from build123d import *

# Parameters (mm, degrees)
SKETCH1_W           = 35
SKETCH1_H           = 35
BOSS_EXTRUDE2_DEPTH = 20
SKETCH2_W           = 35
SKETCH2_H           = 10
BOSS_EXTRUDE3_DEPTH = 20
SKETCH3_W           = 35
SKETCH3_H           = 35
BOSS_EXTRUDE4_DEPTH = 5
CUT_EXTRUDE1_REACH  = 53.357
SKETCH4_R           = 1.5


with BuildPart() as part:
    # Sketch1 → Boss-Extrude2 (new body)
    with BuildSketch(Plane(origin=(0, 0, 0), x_dir=(1, 0, 0), z_dir=(0, 1, 0))):
        Rectangle(SKETCH1_W, SKETCH1_H)
    extrude(amount=BOSS_EXTRUDE2_DEPTH)

    # Sketch2 → Boss-Extrude3 (add)
    with BuildSketch(Plane(origin=(0, 20, 0), x_dir=(1, 0, 0), z_dir=(0, 1, 0))):
        Rectangle(SKETCH2_W, SKETCH2_H)
    extrude(amount=BOSS_EXTRUDE3_DEPTH)

    # Sketch3 → Boss-Extrude4 (add)
    with BuildSketch(Plane(origin=(0, 40, 0), x_dir=(1, 0, 0), z_dir=(0, 1, 0))):
        Rectangle(SKETCH3_W, SKETCH3_H)
    extrude(amount=BOSS_EXTRUDE4_DEPTH)

    # Sketch4 → Cut-Extrude1 (cut, up to next)
    with BuildSketch(Plane(origin=(0, 45, 0), x_dir=(1, 0, 0), z_dir=(0, 1, 0)), mode=Mode.PRIVATE) as cut_extrude1_sk1:
        with Locations(Location((-14.5, 14.5, 0), (0, 0, 270))):
            Circle(SKETCH4_R)
    cut_extrude1_tool1 = extrude(cut_extrude1_sk1.sketch, amount=-CUT_EXTRUDE1_REACH, mode=Mode.PRIVATE) & part.part
    # Sketch4 → Cut-Extrude1 (cut, up to next)
    with BuildSketch(Plane(origin=(0, 45, 0), x_dir=(1, 0, 0), z_dir=(0, 1, 0)), mode=Mode.PRIVATE) as cut_extrude1_sk2:
        with Locations(Location((14.5, 14.5, 0), (0, 0, 270))):
            Circle(SKETCH4_R)
    cut_extrude1_tool2 = extrude(cut_extrude1_sk2.sketch, amount=-CUT_EXTRUDE1_REACH, mode=Mode.PRIVATE) & part.part
    # Sketch4 → Cut-Extrude1 (cut, up to next)
    with BuildSketch(Plane(origin=(0, 45, 0), x_dir=(1, 0, 0), z_dir=(0, 1, 0)), mode=Mode.PRIVATE) as cut_extrude1_sk3:
        with Locations(Location((14.5, -14.5, 0), (0, 0, 270))):
            Circle(SKETCH4_R)
    cut_extrude1_tool3 = extrude(cut_extrude1_sk3.sketch, amount=-CUT_EXTRUDE1_REACH, mode=Mode.PRIVATE) & part.part
    # Sketch4 → Cut-Extrude1 (cut, up to next)
    with BuildSketch(Plane(origin=(0, 45, 0), x_dir=(1, 0, 0), z_dir=(0, 1, 0)), mode=Mode.PRIVATE) as cut_extrude1_sk4:
        with Locations(Location((-14.5, -14.5, 0), (0, 0, 270))):
            Circle(SKETCH4_R)
    cut_extrude1_tool4 = extrude(cut_extrude1_sk4.sketch, amount=-CUT_EXTRUDE1_REACH, mode=Mode.PRIVATE) & part.part
    add(cut_extrude1_tool1.solids().sort_by_distance((-14.5, 45, -14.5))[0], mode=Mode.SUBTRACT)
    add(cut_extrude1_tool2.solids().sort_by_distance((14.5, 45, -14.5))[0], mode=Mode.SUBTRACT)
    add(cut_extrude1_tool3.solids().sort_by_distance((14.5, 45, 14.5))[0], mode=Mode.SUBTRACT)
    add(cut_extrude1_tool4.solids().sort_by_distance((-14.5, 45, 14.5))[0], mode=Mode.SUBTRACT)


solid = part.part
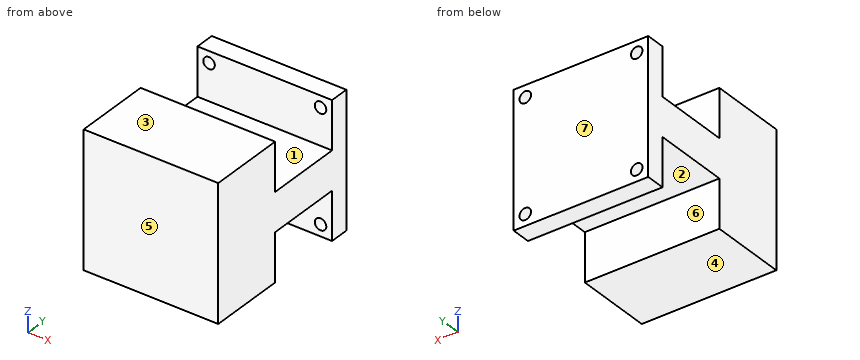
Work out the finished part from the listing and answer in its coordinate system (mm). Face numbers are marked on the shaded views. A direction names the side the tool comes from. Give positions to 0.01 mm unless a question says otherwise; leave off trailing zeros. Order: outer loops, then holes, each group sorted by start corner. A loop starts at its lowest first (then second) coordinate and runs counter-clockwise, first axis right, second up. Notation, with made-up numbers: (74.5, 85.25) - (110.5, 85.25) arc R9 cw to (110.5, 99.25) - close; hole circle Ø9 at (-38.5, -17.5). An arc over 180 degrees is marked (long way). Answer as CSV lines item,"result". Start each with the question number.
Q1. The mould has two halves that part along Y. Classify the marked faces 4, 5, 6 and 7: +Y half, -Y half, draft (parallel to the pull), parting line (faces both ways), or undercut.
Q2. The part is cut by section C-C (z = -14.5). Write down the section's boundary in (x, y), then the cut area to 3 significant figures.
Q3. Find the intervals of material crossed by L1, parallel to X at y = 43.15, z = 14.5; L2, parallel to Y at x = -6, z = -11.5; L3, parallel to X at y = 43, z = -14, in increasing order. Write a range as [from, to].
Q4. The part is cut by section B-B (x = 14.5). Write down the section's boundary in (y, z), then the cut area to 4 significant figures.
Q5. Given pin 1 Ø6 at (x, y) = (4, 29.5) entering from +Z; pin 2 Ø2.5 at (x, z) = (14.5, -14.5) entering from +Y; pin 3 Ø4 at (y, z) = (37, -10) entering from -X, each flat-ended and moving along its own axis, determine where each tip first touches the part or whether it passes through.
Q6. The part is cut by section D-D (x = -12). Write down the section's boundary in (y, z), then the cut area to 4 significant figures.
Q7. The part is cut by section A-A (z = -10). Write down the section's boundary in (x, y).
Q8. For the marked faces 1, 2 and 3, determine the directions among +Z, -Z, +X, -X, +Y, -Y from which every point of the face is accessible in a straight line to the end or side of a thin tool.
Check result:
1,face 4,"draft"
1,face 5,"-Y half"
1,face 6,"undercut"
1,face 7,"+Y half"
2,outline,"(-17.5, 0) - (17.5, 0) - (17.5, 20) - (-17.5, 20) - close; (-17.5, 40) - (-16, 40) - (-16, 45) - (-17.5, 45) - close; (-13, 40) - (13, 40) - (13, 45) - (-13, 45) - close; (16, 40) - (17.5, 40) - (17.5, 45) - (16, 45) - close"
2,area,"845 mm²"
3,L1,"x = [-17.5, -16], [-13, 13], [16, 17.5]"
3,L2,"y = [0, 20], [40, 45]"
3,L3,"x = [-17.5, -15.91], [-13.09, 13.09], [15.91, 17.5]"
4,outline,"(0, -17.5) - (20, -17.5) - (20, -5) - (40, -5) - (40, -13) - (45, -13) - (45, 13) - (40, 13) - (40, 5) - (20, 5) - (20, 17.5) - (0, 17.5) - close; (40, -17.5) - (45, -17.5) - (45, -16) - (40, -16) - close; (40, 16) - (45, 16) - (45, 17.5) - (40, 17.5) - close"
4,area,"1,045 mm²"
5,pin 1,"stops at z = 5"
5,pin 2,"stops at y = 20"
5,pin 3,"passes through"
6,outline,"(0, -17.5) - (20, -17.5) - (20, -5) - (40, -5) - (40, -17.5) - (45, -17.5) - (45, 17.5) - (40, 17.5) - (40, 5) - (20, 5) - (20, 17.5) - (0, 17.5) - close"
6,area,"1,075 mm²"
7,outline,"(-17.5, 0) - (17.5, 0) - (17.5, 20) - (-17.5, 20) - close; (-17.5, 40) - (17.5, 40) - (17.5, 45) - (-17.5, 45) - close"
8,face 1,"+Z, +X, -X"
8,face 2,"-Z, +X, -X"
8,face 3,"+Z, +X, -X, +Y, -Y"
